For this review, take the finished solid that the model builds, in its own axes (mm). Face numbers are marked on the shaded views. A direction names the side the tool comes from. Round coordinates to 2 decimals unless told otherwise and drop trailing zeros. Write each loop counter-clockwise with the first axis right and the second up, starting at its lowest first coordinate (ties: lowest second). Pieces come first, ordered by that corner, then holes. Notation, with made-up numbers: M 19,86 L 32,86 A21 cw 32,103 Z; hole C 88,1 d3. An arc over 180 degrees is marked long. Write each question's results on one line, items separated by ' | '. Start each with the question number.
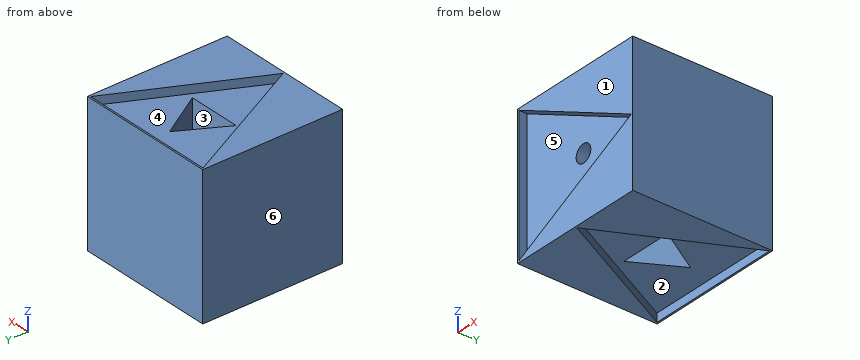
```python
from build123d import *

# Parameters (mm, degrees)
F0_W     = 50
F0_H     = 50
F1_DEPTH = 25
F2_DEPTH = 22
F4_DEPTH = 48
F5_R     = 3.175
F6_DEPTH = 38.77081
F8_DEPTH = 3


with BuildPart() as f1:
    # F0 (on Top) → F1 (new body, symmetric)
    with BuildSketch(Plane.XY):
        with Locations((4.845758, 7.249413)):
            Rectangle(F0_W, F0_H)
        Polygon((4.845758, -17.152166), (-19.555818, 31.650989), (29.247334, 31.650989), align=None, mode=Mode.SUBTRACT)
    extrude(amount=F1_DEPTH, both=True)

    # F0 (on Top) → F2 (join, symmetric)
    with BuildSketch(Plane.XY):
        Polygon((29.247334, 31.650989), (-19.555818, 31.650989), (4.845758, -17.152166), align=None)
    extrude(amount=F2_DEPTH, both=True)

    # F3 (on face) → F4 (cut)
    with BuildSketch(Plane(origin=(0, 0, -22), x_dir=(1, 0, 0), z_dir=(0, 0, -1))):
        Polygon((-4.337861, -7.249412), (4.845758, -23.51713), (14.662139, -7.249412), align=None)
    extrude(amount=-F4_DEPTH, mode=Mode.SUBTRACT)

    # F5 (on face) → F6 (cut)
    with BuildSketch(Plane.XZ.offset(17.750587)):
        with Locations((4.845758, 0)):
            Circle(F5_R)
    extrude(amount=-F6_DEPTH, mode=Mode.SUBTRACT)

    # F7 (on face) → F8 (cut)
    with BuildSketch(Plane.XZ.offset(17.750587)):
        Polygon((29.247338, 0), (-19.555822, 24.40158), (-19.555822, -24.40158), align=None)
    extrude(amount=-F8_DEPTH, mode=Mode.SUBTRACT)


solid = f1.part
```
Item 1: Mouldability with a two-part tool opening along Y and no side actions: class the marked faces 4, 5 and 6 as pulls with the +Y half, pulls with the -Y half, needs draft (parallel to the pull), parting line crosses it, or undercut.
Item 2: Insertion check: P1, Ø2, axis at x = -8, z = 13.5, coming from the -Y side; P2, Ø0.5, axis at x = 7, z = 0.5, coming from the -Y side; P3, Ø24.5, axis at x = 8, z = -1.5, coming from the -Y side; P4, Ø5, axis at x = -5, y = 22, coming from the -Z side. Each pin has a flat end and moves straight along its axis. Give the tip position at first contact, or say it passes through.
Item 3: For the marked faces 1, 2 and 3, list the 3-axis set-ups (+Z, -Z, +X, -X, +Y, -Y) from which the entire face can be reached by the end or side of a thin tool; tool diameter is ignored.
Item 4: We need section B-B on z = -20. State the section outline as (x, y) points, then the cut area to 3 significant figures.
Item 5: We need section C-C on y = 25. State the section outline as (x, z) points.
Item 6: We need section D-D on z = -8. State the section outline as (x, y) points.
Item 7: For probe 1 along Z at (x, y) = (5, -3); probe 2 along Z at (x, y) = (-1.5, -0.5); probe 3 along Y at (x, z) = (-11.5, 5), list the stretches that pass through material, from the lowest coordinate up.
Item 8: We need section A-A on x = 12.5. State the section outline as (y, z) points.
Numbers:
1) face 4: undercut | face 5: pulls with the -Y half | face 6: needs draft
2) P1: stops at y = -14.75 | P2: stops at y = 21.02 | P3: stops at y = -17.75 | P4: stops at z = -22
3) face 1: +Z, -Z, +X, -X, -Y | face 2: -Z | face 3: +Z, -Z
4) outline: M -20.15,-17.75 L -19.56,-17.75 L -19.56,-14.75 L -10.75,-14.75 L -10.75,-17.75 L 29.85,-17.75 L 29.85,32.25 L -20.15,32.25 Z; hole M -4.34,7.25 L 14.66,7.25 L 4.85,23.52 Z | area: 2,320 mm^2
5) outline: M -20.15,-25 L -16.23,-25 L -16.23,-22 L 25.92,-22 L 25.92,-25 L 29.85,-25 L 29.85,25 L 25.92,25 L 25.92,22 L -16.23,22 L -16.23,25 L -20.15,25 Z
6) outline: M -20.15,-17.75 L -19.56,-17.75 L -19.56,-14.75 L 13.25,-14.75 L 13.25,-17.75 L 29.85,-17.75 L 29.85,32.25 L -20.15,32.25 Z; hole M -4.34,7.25 L 14.66,7.25 L 4.85,23.52 Z
7) probe 1: z = -22 to -3.17, 3.17 to 22 | probe 2: z = -22 to 22 | probe 3: y = -14.75 to 32.25
8) outline: M -17.75,-25 L -1.84,-25 L -1.84,-22 L 7.25,-22 L 7.25,22 L -1.84,22 L -1.84,25 L -17.75,25 L -17.75,8.37 L -14.75,8.37 L -14.75,-8.37 L -17.75,-8.37 Z; M 10.83,-22 L 31.65,-22 L 31.65,-25 L 32.25,-25 L 32.25,25 L 31.65,25 L 31.65,22 L 10.83,22 Z
